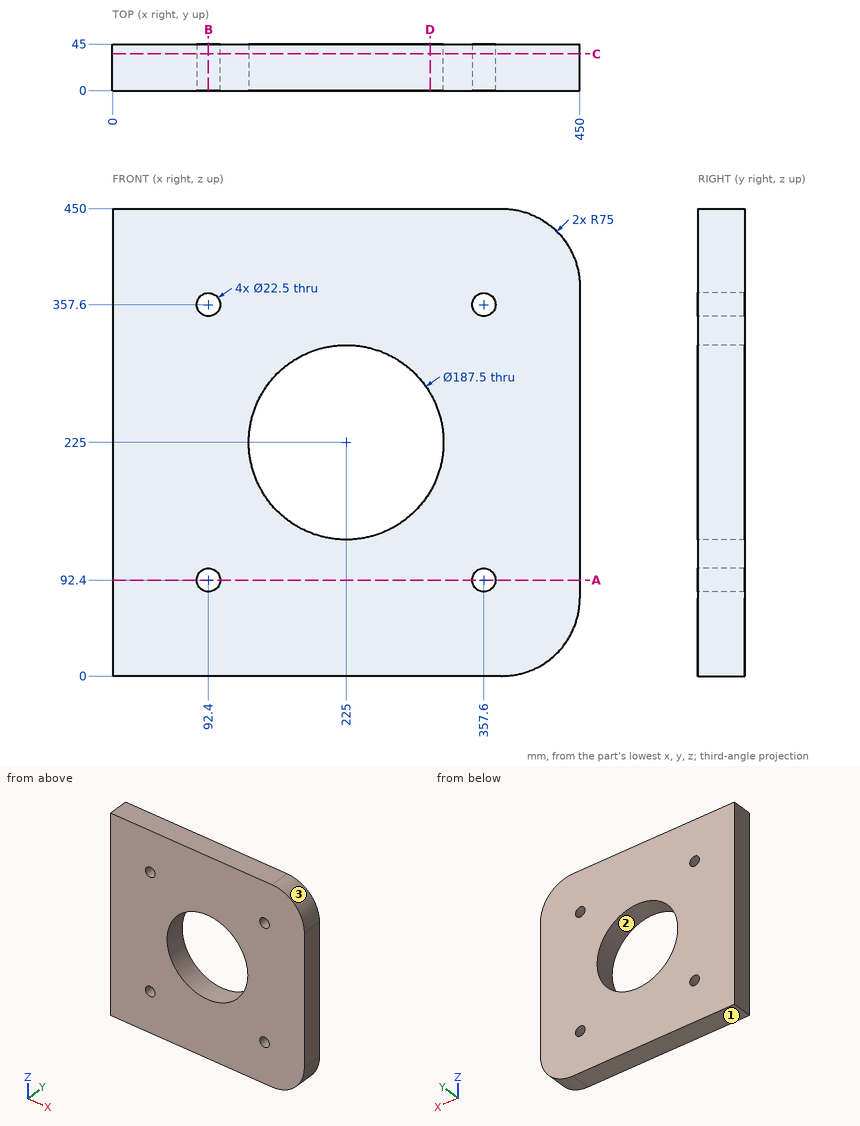
Here's the drawing with two shaded views (mm, measured from the low corner). I have some questions. Give positions to 0.01 mm unless a question says otherwise; leave off trailing zeros. Order: outer loops, then holes, each group sorted by start corner. A loop starts at its lowest first (then second) coordinate and runs counter-clockwise, first axis right, second up. Notation, with made-up numbers: (27.5, 87) - (47.5, 87) arc R33 ccw to (47.5, 122) - close; hole circle Ø11 at (42.5, 24). An arc over 180 degrees is marked (long way). Use a Markdown table: item, result. Add a question column.
Q1. If we mould it in two halves opening along Z, with no side actions, what happens to the marked faces 1, 2 and 3? For each: released by +Z, released by -Z, zero draft, split by the parting line, or undercut.
Q2. I'm going to push a flat-ended pin straight in: pin 1 (12 mm diameter, centred on x = 309, z = 310.5, fed in from -Y). Where does the tip first touch, or does it pass through?
Q3. Please list where these lines run through material, in increasing order: line 1 along Z through (x, y) = (92, 24); line 2 along X through (y, z) = (27, 357.6); line 3 along Z through (x, y) = (225, 33).
Q4. If we section it at D-D on x = 306: Write out the boundary of the cut face in (y, z).
Q5. If we section it at B-B on x = 92.4: Write out the boundary of the cut face in (y, z).
Q6. If we section it at C-C on y = 35.5: Write out the boundary of the cut face in (x, z), plus the area to 3 significant figures.
Q7. If we section it at A-A on z = 92.4: Write out the boundary of the cut face in (x, y), plus the area to 3 significant figures.
Answers follow:
| question | item | result |
|---|---|---|
| 1 | face 1 | released by -Z |
| 1 | face 2 | undercut |
| 1 | face 3 | released by +Z |
| 2 | pin 1 | stops at y = 0 |
| 3 | line 1 | z = 0 to 81.16, 103.64 to 346.36, 368.84 to 450 |
| 3 | line 2 | x = 0 to 81.15, 103.65 to 346.35, 368.85 to 450 |
| 3 | line 3 | z = 0 to 131.25, 318.75 to 450 |
| 4 | outline | (0, 0) - (45, 0) - (45, 177.8) - (0, 177.8) - close; (0, 272.2) - (45, 272.2) - (45, 450) - (0, 450) - close |
| 5 | outline | (0, 0) - (45, 0) - (45, 81.15) - (0, 81.15) - close; (0, 103.65) - (45, 103.65) - (45, 346.35) - (0, 346.35) - close; (0, 368.85) - (45, 368.85) - (45, 450) - (0, 450) - close |
| 6 | outline | (0, 0) - (375, 0) arc R75 ccw to (450, 75) - (450, 375) arc R75 ccw to (375, 450) - (0, 450) - close; hole circle Ø22.5 at (92.4, 92.4); hole circle Ø22.5 at (92.4, 357.6); hole circle Ø187.5 at (225, 225); hole circle Ø22.5 at (357.6, 92.4); hole circle Ø22.5 at (357.6, 357.6) |
| 6 | area | 171,000 mm^2 |
| 7 | outline | (0, 0) - (81.15, 0) - (81.15, 45) - (0, 45) - close; (103.65, 0) - (346.35, 0) - (346.35, 45) - (103.65, 45) - close; (368.85, 0) - (450, 0) - (450, 45) - (368.85, 45) - close |
| 7 | area | 18,200 mm^2 |
